Could you check a few things on this model? Use its own coordinates, in mm. Coordinates: 2 decimals unless noted, no trailing zeros. Loops run counter-clockwise (first coordinate to the right, second up) from the corner with the lowest first, then second, coordinate; pieces in that order, holes last.
from build123d import *

# Parameters (mm, degrees)
SKETCH1_R           = 4.445
BOSS_EXTRUDE1_DEPTH = 2.54
FILLET1_R           = 10.16


with BuildPart() as part:
    # Sketch1 → Boss-Extrude1 (new body)
    with BuildSketch(Plane.XY):
        with BuildLine():
            Line((0, -10.3124), (0, -142.24))
            Line((0, -142.24), (142.24, -142.24))
            Line((142.24, -142.24), (142.24, 0))
            Line((142.24, 0), (10.3124, 0))
            ThreePointArc((10.3124, 0), (-7.29196797, 7.29196797), (0, -10.3124))
        make_face()
        Circle(SKETCH1_R, mode=Mode.SUBTRACT)
    extrude(amount=BOSS_EXTRUDE1_DEPTH)

    # Fillet1
    fillet1_edges = [part.edges().sort_by_distance(p)[0] for p in [
        (0, -10.3124, 1.27),
        (10.3124, 0, 1.27),
    ]]
    fillet(fillet1_edges, radius=FILLET1_R)


solid = part.part
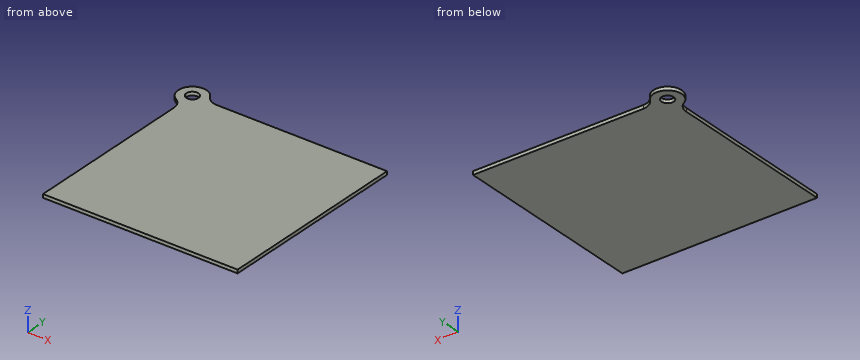
1) If I drill on L1, parallel to X at y = -79.5, z = 1.75; L2, parallel to Y at x = 89, z = 0.55; L3, parallel to X at y = 2, z = 0.35, over which ranges is the centre line in solid material (lowest first)?
2) Imagine slicing it at B-B on y = -2. List the corners of the cut face in (x, z) for me, plus the area to 3 significant figures.
3) Will this pin go through, and if not, where does the flat tip stop? pin 1 (0.8 mm diameter, centred on y = -95, z = 1.5, fed in from -X).
4) Imagine slicing it at D-D on y = -47. List the corners of the cut face in (x, z) for me.
5) Imagine slicing it at C-C on x = 45.5. List the corners of the cut face in (y, z) for me.
6) Imagine slicing it at A-A on z = 1.7. List the corners of the cut face in (x, y) for me (3 decimals).
Solved:
1. L1: x = 0 to 142.24
1. L2: y = -142.24 to 0
1. L3: x = -10.12 to -3.97, 3.97 to 11.72
2. outline: (-10.12, 0) - (-3.97, 0) - (-3.97, 2.54) - (-10.12, 2.54) - close; (3.97, 0) - (142.24, 0) - (142.24, 2.54) - (3.97, 2.54) - close
2. area: 367 mm2
3. pin 1: stops at x = 0
4. outline: (0, 0) - (142.24, 0) - (142.24, 2.54) - (0, 2.54) - close
5. outline: (-142.24, 0) - (0, 0) - (0, 2.54) - (-142.24, 2.54) - close
6. outline: (-5.118, -8.953) arc R10.16 cw to (0, -17.773) - (0, -142.24) - (142.24, -142.24) - (142.24, 0) - (17.773, 0) arc R10.16 cw to (8.953, 5.118) arc R10.312 ccw (long way) to start; hole circle Ø8.89 at (0, 0)
